Build history of the part. All positions in model axes, mm. Give positions to 0.01 mm unless a question says otherwise; leave off trailing zeros.
from build123d import *

# Parameters (mm, degrees)
ESQUISSE1_W             = 20
ESQUISSE1_H             = 20
ESQUISSE1_R             = 1.5
BOSS_EXTRU_1_DEPTH      = 300
CONG_1_R                = 2
ESQUISSE2_W             = 8
ESQUISSE2_H             = 1
ESQUISSE2_W_2           = 1
ESQUISSE2_H_2           = 8
ENL_V_MAT_EXTRU_1_DEPTH = 302.330383466


with BuildPart() as part:
    # Esquisse1 → Boss.-Extru.1 (new body)
    with BuildSketch(Plane.XY):
        with Locations((-10, 10)):
            Rectangle(ESQUISSE1_W, ESQUISSE1_H)
        with Locations((-10, 10)):
            Circle(ESQUISSE1_R, mode=Mode.SUBTRACT)
        with BuildLine():
            Line((-19, 18.2), (-12.144004756, 11.285785211))
            ThreePointArc((-12.144004756, 11.285785211), (-12.499292367, 10.059478285), (-12.20274135, 8.817658871))
            Line((-12.20274135, 8.817658871), (-19, 1.8))
            Line((-19, 1.8), (-19, 18.2))
        make_face(mode=Mode.SUBTRACT)
        with BuildLine():
            Line((-18.2, 1), (-1.8, 1))
            Line((-1.8, 1), (-8.678082464, 7.878082464))
            ThreePointArc((-8.678082464, 7.878082464), (-10.078866736, 7.501244302), (-11.453098741, 7.965668648))
            Line((-11.453098741, 7.965668648), (-18.2, 1))
        make_face(mode=Mode.SUBTRACT)
        with BuildLine():
            Line((-1, 18.2), (-1, 1.8))
            Line((-1, 1.8), (-7.878082464, 8.678082464))
            ThreePointArc((-7.878082464, 8.678082464), (-7.5, 10), (-7.878082464, 11.321917536))
            Line((-7.878082464, 11.321917536), (-1, 18.2))
        make_face(mode=Mode.SUBTRACT)
        with BuildLine():
            Line((-11.357461746, 12.099356475), (-18.2, 19))
            Line((-18.2, 19), (-1.8, 19))
            Line((-1.8, 19), (-8.678082464, 12.121917536))
            ThreePointArc((-8.678082464, 12.121917536), (-10.021049895, 12.499911379), (-11.357461746, 12.099356475))
        make_face(mode=Mode.SUBTRACT)
    extrude(amount=BOSS_EXTRU_1_DEPTH)

    # Congé1
    cong_1_edges = [part.edges().sort_by_distance(p)[0] for p in [
        (0, 0, 150),
        (-20, 0, 150),
        (-20, 20, 150),
        (0, 20, 150),
    ]]
    fillet(cong_1_edges, radius=CONG_1_R)

    # Esquisse2 → Enlèv. mat.-Extru.1 (cut, through all)
    with BuildSketch(Plane.XY.offset(300)):
        with Locations((-10, 19.5)):
            Rectangle(ESQUISSE2_W, ESQUISSE2_H)
        with Locations((-19.5, 10)):
            Rectangle(ESQUISSE2_W_2, ESQUISSE2_H_2)
        with Locations((-10, 0.5)):
            Rectangle(ESQUISSE2_W, ESQUISSE2_H)
        with Locations((-0.5, 10)):
            Rectangle(ESQUISSE2_W_2, ESQUISSE2_H_2)
    extrude(amount=-ENL_V_MAT_EXTRU_1_DEPTH, mode=Mode.SUBTRACT)


solid = part.part
1. Drop flat-ended pins along their axis: pin 1 (8 mm diameter, centred on x = -9.5, y = 7, fed in from +Z); pin 2 (1.1 mm diameter, centred on y = 0.5, z = 116, fed in from -X); pin 3 (4 mm diameter, centred on y = 11.5, z = 112, fed in from +X); pin 4 (3 mm diameter, centred on y = 10.5, z = 71.5, fed in from -X). Give the stop position or say it passes through.
2. Drill centre lines: line 1 along Y through (x, z) = (-10, 191); line 2 along Y through (x, z) = (-3, 268.5); line 3 along X through (y, z) = (16, 150). Where is each one in solid material? Low to high.
3. Mould opens along Y. For faces 1 (the face through (-12, 10, 0)), 2 (the face through (-5.2, 15.6, 147.9)) say: pulls with the +Y half, pulls with the -Y half, needs draft (parallel to the pull), parting line crosses it, or undercut.
Outcome:
1. pin 1: stops at z = 300
1. pin 2: stops at x = -19.76
1. pin 3: stops at x = -5.7
1. pin 4: stops at x = -12.85
2. line 1: y = 7.5 to 8.5, 11.5 to 12.5
2. line 2: y = 0 to 1, 2.2 to 3.8, 16.2 to 17.8, 19 to 20
2. line 3: x = -20 to -19, -16.82 to -15.23, -4.8 to -3.2, -1 to 0
3. face 1: needs draft
3. face 2: undercut
